The model under review builds one solid part; all positions refer to its coordinate system, in mm. A direction names the side the tool comes from. Give positions to 0.01 mm unless a question says otherwise; leave off trailing zeros. Loops run counter-clockwise (first coordinate to the right, second up) from the corner with the lowest first, then second, coordinate; pieces in that order, holes last. Notation, with made-up numbers: M 68.5,46 L 74.5,46 A10 ccw 74.5,64 Z; hole C -17,52 d5. An arc over 180 degrees is marked long. One line per item, written item: value. Start each with the question number.
Q1. We need section B-B on x = -86. Write out the cut boundary in (y, z), plus the area to 3 significant figures.
Q2. To check wall thickness, follow line 1 along Z through (x, y) = (-170.5, 0.5). State the ranges of the line that lie inside material, in increasing order. Write a range as from..to.
Q3. Mouldability with a two-part tool opening along Z and no side actions: class faces 3 (the face through (-4, 6.35, 3)), 4 (the face through (171.003, 3.131, -64.443)) as released by +Z, released by -Z, zero draft, split by the parting line, or undercut.
Q4. For faces 1 (the face through (95.894, 3.131, -64.641)), 2 (the face through (-4, 0, 3)), list the 3-axis set-ups (+Z, -Z, +X, -X, +Y, -Y) from which the entire face can be reached by the end or side of a thin tool; tool diameter is ignored.
Q5. We need section A-A on z = 28. Give the number of separate pieces and of enclosed holes in the cut face, plus the area to 3 significant figures.
```python
from build123d import *

# Parameters (mm, degrees)
F0_W     = 520.7
F0_H     = 406.4
F0_W_2   = 179.3875
F0_H_2   = 314.325
F1_DEPTH = 6.35


with BuildPart() as f1:
    # F0 (on Front) → F1 (new body)
    with BuildSketch(Plane.XZ):
        Rectangle(F0_W, F0_H)
        with Locations((-124.61875, 0)):
            Rectangle(F0_W_2, F0_H_2, mode=Mode.SUBTRACT)
        with BuildLine():
            ThreePointArc((92.075, 39.6875), (95.794744, 48.667756), (104.775, 52.3875))
            Line((104.775, 52.3875), (161.925, 52.3875))
            ThreePointArc((161.925, 52.3875), (170.905256, 48.667756), (174.625, 39.6875))
            Line((174.625, 39.6875), (174.625, -55.5625))
            ThreePointArc((174.625, -55.5625), (170.905256, -64.542756), (161.925, -68.2625))
            Line((161.925, -68.2625), (104.775, -68.2625))
            ThreePointArc((104.775, -68.2625), (95.794744, -64.542756), (92.075, -55.5625))
            Line((92.075, -55.5625), (92.075, 39.6875))
        make_face(mode=Mode.SUBTRACT)
    extrude(amount=-F1_DEPTH)


solid = f1.part
```
Solved:
1. outline: M 0,-203.2 L 6.35,-203.2 L 6.35,-157.16 L 0,-157.16 Z; M 0,157.16 L 6.35,157.16 L 6.35,203.2 L 0,203.2 Z
1. area: 585 mm2
2. line 1: -203.2..-157.16, 157.16..203.2
3. face 3: zero draft
3. face 4: undercut
4. face 1: +Y, -Y
4. face 2: +Z, -Z, +X, -X, -Y
5. separate pieces: 3
5. enclosed holes: 0
5. area: 1,640 mm2
